Here's how the part is built. I have some questions about the finished solid (model axes, mm). Round coordinates to 2 decimals unless told otherwise and drop trailing zeros. Write each loop counter-clockwise with the first axis right and the second up, starting at its lowest first coordinate (ties: lowest second). Pieces come first, ordered by that corner, then holes. Notation, with made-up numbers: (-19, 82) -> (11, 82) arc R18 ccw to (11, 88) -> close; hole circle Ø8 at (4.25, 36.5). An arc over 180 degrees is marked (long way). Put each result on its own line as item: value. Start each with the question number.
1) I want a section at A-A, the plane x = 0.2. Give the number of separate pieces and of enclosed holes in the cut face, then the cut area to 3 significant figures.
2) If I drill on line 1 along Z through (x, y) = (-0.2, 15); line 2 along Z through (x, y) = (0.2, 0); line 3 along Z through (x, y) = (0.3, 20), over which ranges is the centre line in solid material (lowest first)? Write a range as [from, to].
3) I want a section at B-B, the plane y = -10. List the corners of the cut face in (x, z) for me.
4) Will these pins go through, and if not, where does the flat tip stop? P1, Ø4, axis at y = 10.26, z = -260.76, coming from the +X side; P2, Ø5, axis at y = 14.5, z = -265, coming from the -X side.
Autodesk Inventor part; units mm, degrees
ref_plane "YZ Plane" through (0, 0, 0) normal (1, 0, 0) x (0, 1, 0)
ref_plane "XZ Plane" through (0, 0, 0) normal (0, 1, 0) x (-1, 0, 0)
ref_plane "XY Plane" through (0, 0, 0) normal (0, 0, 1) x (1, 0, 0)
sketch "スケッチ1" plane through (0, 0, 0) normal (1, 0, 0) x (0, 1, 0)
  line L0 (-24.5, 275) -> (24.5, 275)
  line L1 (24.5, 275) -> (24.5, -275)
  line L2 (24.5, -275) -> (-24.5, -275)
  line L3 (-24.5, -275) -> (-24.5, 275)
  line L4 (-24.5, 275) -> (24.5, -275) construction
  line L5 (24.5, 275) -> (-24.5, -275) construction
  point P0 (0, 0)
  dimension "d0" = 49
  dimension "d1" = 550
extrude "プレート1" add sketch "スケッチ1" along normal mid plane 1
sketch "スケッチ3" plane through (0.5, 0, 0) normal (1, 0, 0) x (0, 0, -1)
  circle A0 centre (265, 14.5) radius 6
  line L0 (275, 24.5) -> (275, -24.5)
  line L1 (-275, 24.5) -> (275, 24.5)
  point P0 (0, 0)
  point P1 (269.2426, 18.7426)
  point P2 (260.7574, 18.7426)
  point P3 (260.7574, 10.2574)
  point P4 (269.2426, 10.2574)
  dimension "d13" = 12
  dimension "d14" = 10
  dimension "d15" = 10
  dimension "d18" = 360
  dimension "d30" = 0
hole "穴2" at (0.5, 18.7426, -269.2426) at (0.5, 18.7426, -260.7574) at (0.5, 10.2574, -260.7574) at (0.5, 10.2574, -269.2426) direction (-1, 0, 0) diameter 3.2 end through all
sketch "スケッチ4" plane through (0.5, 0, 0) normal (1, 0, 0) x (0, 0, -1)
  circle A0 centre (265, 14.5) radius 3.05
  point P0 (0, 0)
  dimension "d27" = 6.1
extrude "押し出し1" cut sketch "スケッチ4" against normal blind 10
sketch "スケッチ5" plane through (0.5, 0, 0) normal (1, 0, 0) x (0, 0, -1)
  line L0 (275, -24.5) -> (236, -24.5)
  line L1 (236, -24.5) -> (236, 4.5)
  line L2 (236, 4.5) -> (275, 4.5)
  line L3 (275, 4.5) -> (275, -24.5)
  line L4 (-275, 24.5) -> (216, 24.5)
  line L5 (216, 24.5) -> (216, 4.5)
  line L6 (216, 4.5) -> (-275, 4.5)
  line L7 (-275, 4.5) -> (-275, 24.5)
  line L8 (275, -24.5) -> (-275, -24.5)
  circle A0 centre (265, 14.5) radius 3.05
  point P0 (0, 0)
  dimension "d35" = 29
  dimension "d36" = 20
  dimension "d40" = 29
  dimension "d41" = 10
extrude "押し出し2" cut sketch "スケッチ5" against normal blind 10 contours L0 L1 L2 L3
fillet "コーナーR2" radius 10 2 edges at (0, 24.5, -275) (0, 4.5, -275)
fillet "コーナーR3" radius 2 3 edges at (0, 4.5, -236) (0, -24.5, -236) (0, -24.5, 275)
equation "\"d25\" = Thickness"
equation "\"d2\" = Thickness"
equation "\"BendRadius\" = Thickness"
equation "\"BendReliefWidth\" = Thickness"
equation "\"BendReliefDepth\" = 0.5 * Thickness"
equation "\"CornerReliefSize\" = 4 * Thickness"
equation "\"MinimumRemnant\" = 2 * Thickness"
equation "\"TransitionRadius\" = BendRadius"
equation "\"JacobiRadiusSize\" = BendRadius"
equation "\"GapSize\" = Thickness"
properties part number "s_carbon_plate5" material "CFRP"
Findings:
1. separate pieces: 1
1. enclosed holes: 5
1. area: 25,700 mm2
2. line 1: z = [-274.99, -268.01], [-261.99, 275]
2. line 2: z = [-236, 275]
2. line 3: z = [-273.35, -270.23], [-268.25, -261.75], [-259.77, 275]
3. outline: (-0.5, -236) -> (0.5, -236) -> (0.5, 275) -> (-0.5, 275) -> close
4. P1: stops at x = 0.5
4. P2: passes through
